Design review of the part shown in the three views and the two pictorial views. Dimensions are in mm from the part's minimum x, y and z. A direction names the side the tool comes from. Round coordinates to 2 decimals unless told otherwise and drop trailing zeros. Loops run counter-clockwise (first coordinate to the right, second up) from the corner with the lowest first, then second, coordinate; pieces in that order, holes last.
1) Mouldability with a two-part tool opening along Y and no side actions: class the marked faces 1, 2 and 3 as pulls with the +Y half, pulls with the -Y half, needs draft (parallel to the pull), parting line crosses it, or undercut.
2) Take a section at B-B (x = 17.5). State the section outline as (y, z) points, then the cut area to 3 significant figures.
3) Take a section at D-D (y = 5). State the section outline as (x, z) points, then the cut area to 3 significant figures.
4) Tool access review of the marked faces 4 and 5: name each direction out of +Z, -Z, +X, -X, +Y, -Y from which nothing blocks a thin tool from reaching the whole face with its end or side.
5) Insertion check: pin 1 (1.5 mm diameter, centred on y = 14.5, z = 1, fed in from -X); pin 2 (3 mm diameter, centred on x = 32, y = 25, fed in from -Z). Each pin has a flat end and moves straight along its axis. Give the tip position at first contact, or say it passes through.
6) Take a section at C-C (z = 2.15). State the section outline as (x, y) points.
7) Take a section at A-A (y = 8.25). State the section outline as (x, z) points.
8) Wall thickness on L1, parallel to Y at x = 32, z = 1.65; L2, parallel to Y at x = 13, z = 0.7; L3, parallel to X at y = 13.5, z = 2.5: over which ranges is each line inside the solid? List them lowest first.
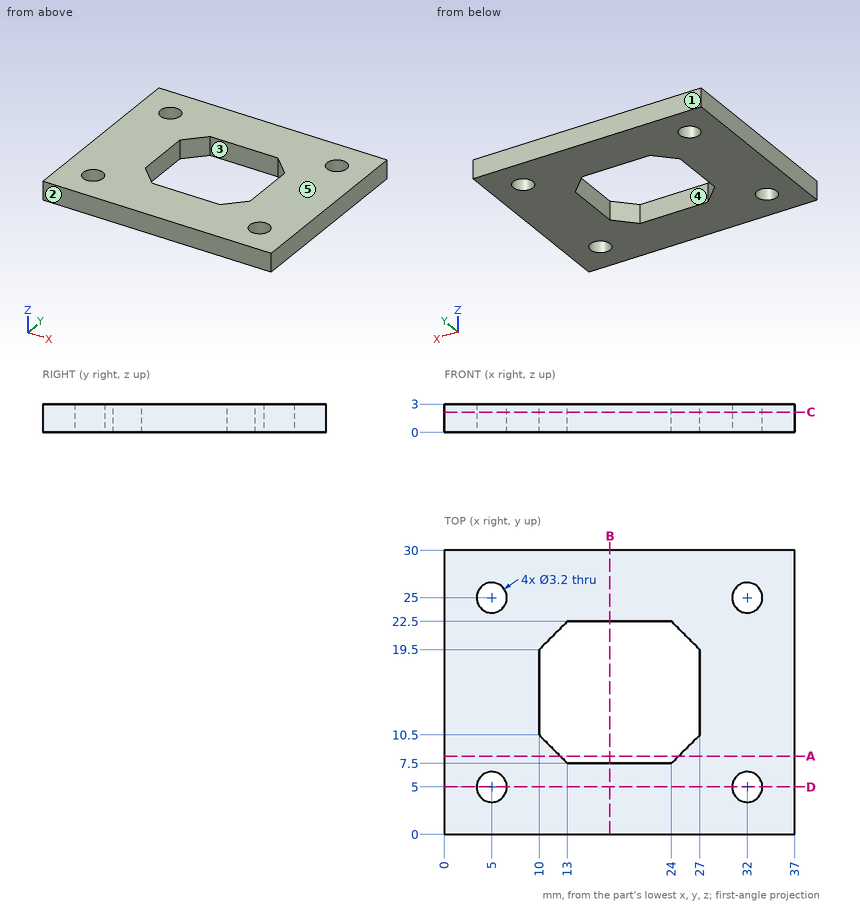
Response:
1. face 1: pulls with the +Y half
1. face 2: pulls with the -Y half
1. face 3: undercut
2. outline: (0, 0) - (7.5, 0) - (7.5, 3) - (0, 3) - close; (22.5, 0) - (30, 0) - (30, 3) - (22.5, 3) - close
2. area: 45.0 mm2
3. outline: (0, 0) - (3.4, 0) - (3.4, 3) - (0, 3) - close; (6.6, 0) - (30.4, 0) - (30.4, 3) - (6.6, 3) - close; (33.6, 0) - (37, 0) - (37, 3) - (33.6, 3) - close
3. area: 91.8 mm2
4. face 4: +Z, -Z
4. face 5: +Z, +X, -X, +Y, -Y
5. pin 1: stops at x = 0
5. pin 2: passes through
6. outline: (0, 0) - (37, 0) - (37, 30) - (0, 30) - close; hole circle Ø3.2 at (5, 5); hole circle Ø3.2 at (5, 25); hole (10, 10.5) - (13, 7.5) - (24, 7.5) - (27, 10.5) - (27, 19.5) - (24, 22.5) - (13, 22.5) - (10, 19.5) - close; hole circle Ø3.2 at (32, 5); hole circle Ø3.2 at (32, 25)
7. outline: (0, 0) - (12.25, 0) - (12.25, 3) - (0, 3) - close; (24.75, 0) - (37, 0) - (37, 3) - (24.75, 3) - close
8. L1: y = 0 to 3.4, 6.6 to 23.4, 26.6 to 30
8. L2: y = 0 to 7.5, 22.5 to 30
8. L3: x = 0 to 10, 27 to 37
